```python
from build123d import *

# Parameters (mm, degrees)
SKETCH11_R          = 3.3672
CUT_EXTRUDE5_DEPTH  = 3.81
SKETCH11_5_R        = 3.3672
CUT_EXTRUDE7_DEPTH  = 7.62
CUT_EXTRUDE8_DEPTH  = 10.16
SKETCH13_R          = 6.35
CUT_EXTRUDE10_DEPTH = 12.192
CHAMFER1_SIZE       = 3.81
CHAMFER2_SIZE       = 6.35
CUT_EXTRUDE11_DEPTH = 9.525


with BuildPart() as part:
    # Sketch2 → Revolve1 (revolve)
    with BuildSketch(Plane(origin=(0, 0, 0), x_dir=(0, 0, -1), z_dir=(1, 0, 0))):
        Polygon((-13.081, 0), (-13.081, 9.525), (-13.081, 12.7), (-9.906, 12.7), (9.906, 12.7), (9.906, 31.75), (13.081, 31.75), (13.081, 0), align=None)
    revolve(axis=Axis((0, 0, -13.081), (0, 0, 1)))

    # Sketch11 → Cut-Extrude5 (cut)
    with BuildSketch(Plane.XY.offset(13.081)):
        with BuildLine():
            ThreePointArc((-6.195622147, -4.226614037), (-3.288572679, -6.740570431), (0.482036294, -7.48449337))
            ThreePointArc((0.482036294, -7.48449337), (-0.337099755, -5.872751112), (-0.749008883, -4.112345522))
            ThreePointArc((-0.749008883, -4.112345522), (-1.832831173, -3.756744587), (-2.78016744, -3.121388955))
            ThreePointArc((-2.78016744, -3.121388955), (-4.421160263, -3.880229865), (-6.195622147, -4.226614037))
        make_face()
        with BuildLine():
            ThreePointArc((7.5, 0), (7.166490288, 2.211654799), (6.195622147, 4.226614037))
            ThreePointArc((6.195622147, 4.226614037), (4.421160263, 3.880229865), (2.78016744, 3.121388955))
            ThreePointArc((2.78016744, 3.121388955), (1.832831173, 3.756744587), (0.749008883, 4.112345522))
            ThreePointArc((0.749008883, 4.112345522), (0.337099755, 5.872751112), (-0.482036294, 7.48449337))
            ThreePointArc((-0.482036294, 7.48449337), (-6.740570431, 3.288572679), (-6.195622147, -4.226614037))
            ThreePointArc((-6.195622147, -4.226614037), (-4.421160263, -3.880229865), (-2.78016744, -3.121388955))
            ThreePointArc((-2.78016744, -3.121388955), (-1.832831173, -3.756744587), (-0.749008883, -4.112345522))
            ThreePointArc((-0.749008883, -4.112345522), (-0.337099755, -5.872751112), (0.482036294, -7.48449337))
            ThreePointArc((0.482036294, -7.48449337), (5.471072665, -5.130045214), (7.5, 0))
        make_face()
        Circle(SKETCH11_R, mode=Mode.SUBTRACT)
        Circle(SKETCH11_R)
        with BuildLine():
            ThreePointArc((2.78016744, 3.121388955), (4.421160263, 3.880229865), (6.195622147, 4.226614037))
            ThreePointArc((6.195622147, 4.226614037), (3.288572679, 6.740570431), (-0.482036294, 7.48449337))
            ThreePointArc((-0.482036294, 7.48449337), (0.337099755, 5.872751112), (0.749008883, 4.112345522))
            ThreePointArc((0.749008883, 4.112345522), (1.832831173, 3.756744587), (2.78016744, 3.121388955))
        make_face()
    extrude(amount=-CUT_EXTRUDE5_DEPTH, mode=Mode.SUBTRACT)

    # Sketch11<5> → Cut-Extrude7 (cut)
    with BuildSketch(Plane.XY.offset(13.081)):
        Circle(SKETCH11_5_R)
    extrude(amount=-CUT_EXTRUDE7_DEPTH, mode=Mode.SUBTRACT)

    # Sketch11<6> → Cut-Extrude8 (cut)
    with BuildSketch(Plane.XY.offset(13.081)):
        with BuildLine():
            ThreePointArc((-6.195622147, -4.226614037), (-3.288572679, -6.740570431), (0.482036294, -7.48449337))
            ThreePointArc((0.482036294, -7.48449337), (-0.337099755, -5.872751112), (-0.749008883, -4.112345522))
            ThreePointArc((-0.749008883, -4.112345522), (-1.832831173, -3.756744587), (-2.78016744, -3.121388955))
            ThreePointArc((-2.78016744, -3.121388955), (-4.421160263, -3.880229865), (-6.195622147, -4.226614037))
        make_face()
        with BuildLine():
            ThreePointArc((2.78016744, 3.121388955), (4.421160263, 3.880229865), (6.195622147, 4.226614037))
            ThreePointArc((6.195622147, 4.226614037), (3.288572679, 6.740570431), (-0.482036294, 7.48449337))
            ThreePointArc((-0.482036294, 7.48449337), (0.337099755, 5.872751112), (0.749008883, 4.112345522))
            ThreePointArc((0.749008883, 4.112345522), (1.832831173, 3.756744587), (2.78016744, 3.121388955))
        make_face()
    extrude(amount=-CUT_EXTRUDE8_DEPTH, mode=Mode.SUBTRACT)

    # Sketch13 → Cut-Extrude10 (cut)
    with BuildSketch(Plane(origin=(0, 0, -13.081), x_dir=(-1, 0, 0), z_dir=(0, 0, -1))):
        Circle(SKETCH13_R)
    extrude(amount=-CUT_EXTRUDE10_DEPTH, mode=Mode.SUBTRACT)

    # Chamfer1
    chamfer1_edges = [part.edges().sort_by_distance(p)[0] for p in [
        (6.35, 0, -0.889),
    ]]
    chamfer(chamfer1_edges, length=CHAMFER1_SIZE)

    # Chamfer2
    chamfer2_edges = [part.edges().sort_by_distance(p)[0] for p in [
        (0, -12.7, -9.906),
    ]]
    chamfer(chamfer2_edges, length=CHAMFER2_SIZE)

    # Sketch14 → Cut-Extrude11 (cut)
    with BuildSketch(Plane.XY.offset(13.081)):
        with BuildLine():
            Line((-7.254714263, 1.902398741), (-12.284649485, 3.221395201))
            ThreePointArc((-12.284649485, 3.221395201), (-12.678861805, -0.732436563), (-11.831978794, -4.614572333))
            Line((-11.831978794, -4.614572333), (-6.987389052, -2.725141142))
            ThreePointArc((-6.987389052, -2.725141142), (-7.487516814, -0.432541277), (-7.254714263, 1.902398741))
        make_face()
        with BuildLine():
            ThreePointArc((-0.732436563, 12.678861805), (-4.614572333, 11.831978794), (-8.045001612, 9.82689926))
            Line((-8.045001612, 9.82689926), (-4.750985204, 5.803286965))
            ThreePointArc((-4.750985204, 5.803286965), (-2.725141142, 6.987389052), (-0.432541277, 7.487516814))
            Line((-0.432541277, 7.487516814), (-0.732436563, 12.678861805))
        make_face()
        with BuildLine():
            ThreePointArc((11.831978794, 4.614572333), (9.82689926, 8.045001612), (6.859894358, 10.68793008))
            Line((6.859894358, 10.68793008), (4.051118716, 6.311769732))
            ThreePointArc((4.051118716, 6.311769732), (5.803286965, 4.750985204), (6.987389052, 2.725141142))
            Line((6.987389052, 2.725141142), (11.831978794, 4.614572333))
        make_face()
        with BuildLine():
            Line((4.750985204, -5.803286965), (8.045001612, -9.82689926))
            ThreePointArc((8.045001612, -9.82689926), (10.68793008, -6.859894358), (12.284649485, -3.221395201))
            Line((12.284649485, -3.221395201), (7.254714263, -1.902398741))
            ThreePointArc((7.254714263, -1.902398741), (6.311769732, -4.051118716), (4.750985204, -5.803286965))
        make_face()
        with BuildLine():
            Line((-4.051118716, -6.311769732), (-6.859894358, -10.68793008))
            ThreePointArc((-6.859894358, -10.68793008), (-3.221395201, -12.284649485), (0.732436563, -12.678861805))
            Line((0.732436563, -12.678861805), (0.432541277, -7.487516814))
            ThreePointArc((0.432541277, -7.487516814), (-1.902398741, -7.254714263), (-4.051118716, -6.311769732))
        make_face()
    extrude(amount=-CUT_EXTRUDE11_DEPTH, mode=Mode.SUBTRACT)


solid = part.part
```
Check sheet for the modelled part. Datum: model origin and axes. Units: mm. A direction names the side the tool comes from. Give positions to 0.01 mm unless a question says otherwise; leave off trailing zeros. Loops run counter-clockwise (first coordinate to the right, second up) from the corner with the lowest first, then second, coordinate; pieces in that order, holes last. Notation, with made-up numbers: M 20,25.5 L 36,25.5 A14 ccw 36,34.5 Z; hole C 65,16 d11. An arc over 180 degrees is marked long. Answer in a Markdown table with one row per item.
1) Cross-section at D-D (x = -20). Enter the section's corners in (y, z).
Solutions:
| item | result |
|---|---|
| outline | M -24.66,-13.08 L 24.66,-13.08 L 24.66,-9.91 L -24.66,-9.91 Z |
2) Cross-section at C-C (z = -6.5). Enter the section's corners in (x, y).
Solutions:
| item | result |
|---|---|
| outline | C 0,0 d31.29; hole C 0,0 d12.7 |
3) Cross-section at B-B (x = -26.5). Enter the section's corners in (y, z).
Solutions:
| item | result |
|---|---|
| outline | M -17.49,-13.08 L 17.49,-13.08 L 17.49,-9.91 L -17.49,-9.91 Z |
4) Thickness scan on line 1 (Y direction, x = 0, z = 7.15); line 2 (Z direction, x = 7, y = -22); line 3 (Y direction, x = 0, z = -7.5). Record the ranges inside material, lowest first.
Solutions:
| item | result |
|---|---|
| line 1 | y = -6.66 to -3.37, 3.37 to 6.66, 7.5 to 12.7 |
| line 2 | z = -13.08 to -9.91 |
| line 3 | y = -16.64 to -6.35, 6.35 to 16.64 |
5) Mould release check, pull along Z, two halves, no side actions. Record for faces 5 (the face through (-6.294, 4.079, 11.203)), 6 (the face through (0.591, -2.66, -1.074)), 7 (the face through (-8, -7, 13.081)): released by +Z, released by -Z, zero draft, split by the parting line, or undercut.
Solutions:
| item | result |
|---|---|
| face 5 | zero draft |
| face 6 | released by -Z |
| face 7 | released by +Z |
6) Depth check by flat-ended pin: pin 1 (12 mm diameter, centred on y = -13.5, z = 2.5, fed in from +X); pin 2 (2 mm diameter, centred on x = -1, y = -5, fed in from +Z); pin 3 (1.3 mm diameter, centred on x = 2, y = 4.5, fed in from +Z). Enter the tip coordinate at first touch or a pass-through.
Solutions:
| item | result |
|---|---|
| pin 1 | stops at x = 10.25 |
| pin 2 | stops at z = 9.27 |
| pin 3 | stops at z = 2.92 |
7) Cross-section at A-A (z = 0.5). Enter the section's corners in (x, y).
Solutions:
| item | result |
|---|---|
| outline | C 0,0 d25.4 |
8) Tool access check on faces 1 (the face through (3, 5, 2.921)), 2 (the face through (0, 0, -0.889)), 3 (the face through (5.475, 8.53, 8.385)), 4 (the face through (-9.44, -3.68, 8.39)). Record the directions out of +Z, -Z, +X, -X, +Y, -Y that give a thin tool (end or side, any length) a straight path to the whole face; none if there is none.
Solutions:
| item | result |
|---|---|
| face 1 | +Z |
| face 2 | -Z |
| face 3 | +Z, +X |
| face 4 | +Z, -X |
